Part print with two shaded views. Sizes in mm from the minimum x, y, z corner. Give positions to 0.01 mm unless a question says otherwise; leave off trailing zeros. Write each loop counter-clockwise with the first axis right and the second up, starting at its lowest first coordinate (ties: lowest second). Pieces come first, ordered by that corner, then holes. Notation, with made-up numbers: (87.5, -31) - (135.5, -31) arc R19 ccw to (135.5, -10) - close; hole circle Ø5 at (62.25, -11.5). An arc over 180 degrees is marked (long way). One line per item, written item: value. Start each with the question number.
(1) Drop a flat-ended pin along its axis: P1, Ø3, axis at x = 44, y = 12, coming from the -Z side. Give the stop position or say it passes through.
(2) Cut at A-A, the plane y = 29. List the corners of the cut face in (x, z).
(3) Cut at D-D, the plane x = 4.5. List the corners of the cut face in (y, z).
(4) Probe L1, parallel to Y at x = 28, z = 0.9; L2, parallel to Y at x = 21, z = 0.45; L3, parallel to X at y = 25, z = 0.2. List the from-to ranges inside material, lowest first.
(5) Cut at B-B, the plane x = 28. List the corners of the cut face in (y, z), and give its area (3 significant figures).
(6) Cut at C-C, the plane y = 40. List the corners of the cut face in (x, z).
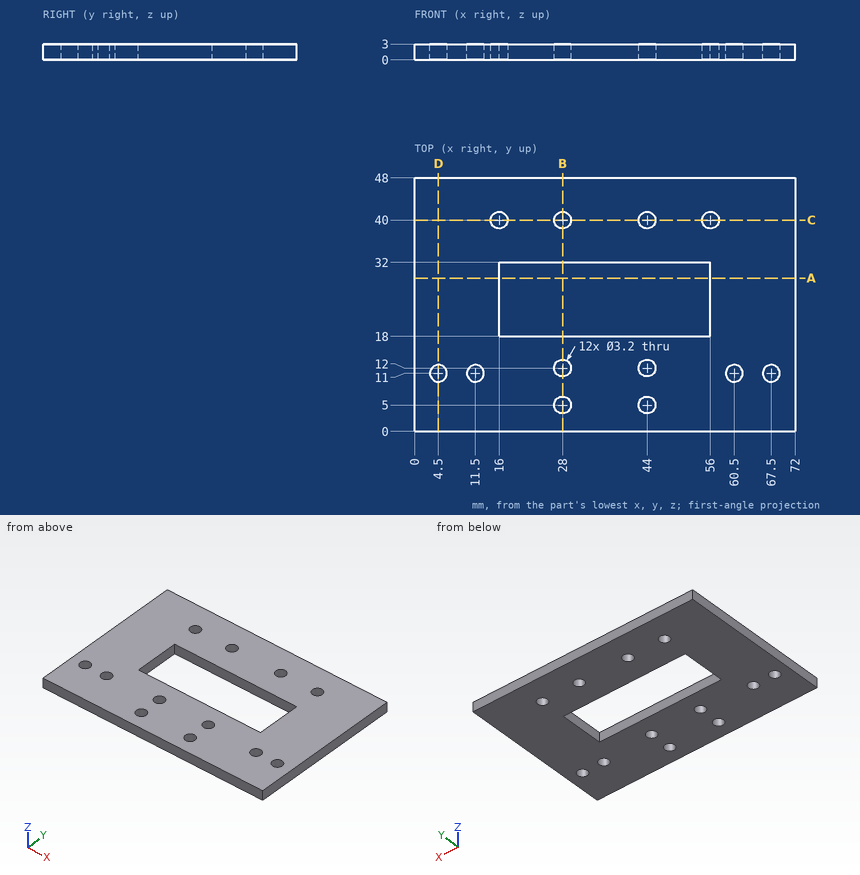
Answers follow:
1. P1: passes through
2. outline: (0, 0) - (16, 0) - (16, 3) - (0, 3) - close; (56, 0) - (72, 0) - (72, 3) - (56, 3) - close
3. outline: (0, 0) - (9.4, 0) - (9.4, 3) - (0, 3) - close; (12.6, 0) - (48, 0) - (48, 3) - (12.6, 3) - close
4. L1: y = 0 to 3.4, 6.6 to 10.4, 13.6 to 18, 32 to 38.4, 41.6 to 48
4. L2: y = 0 to 18, 32 to 48
4. L3: x = 0 to 16, 56 to 72
5. outline: (0, 0) - (3.4, 0) - (3.4, 3) - (0, 3) - close; (6.6, 0) - (10.4, 0) - (10.4, 3) - (6.6, 3) - close; (13.6, 0) - (18, 0) - (18, 3) - (13.6, 3) - close; (32, 0) - (38.4, 0) - (38.4, 3) - (32, 3) - close; (41.6, 0) - (48, 0) - (48, 3) - (41.6, 3) - close
5. area: 73.2 mm²
6. outline: (0, 0) - (14.4, 0) - (14.4, 3) - (0, 3) - close; (17.6, 0) - (26.4, 0) - (26.4, 3) - (17.6, 3) - close; (29.6, 0) - (42.4, 0) - (42.4, 3) - (29.6, 3) - close; (45.6, 0) - (54.4, 0) - (54.4, 3) - (45.6, 3) - close; (57.6, 0) - (72, 0) - (72, 3) - (57.6, 3) - close
